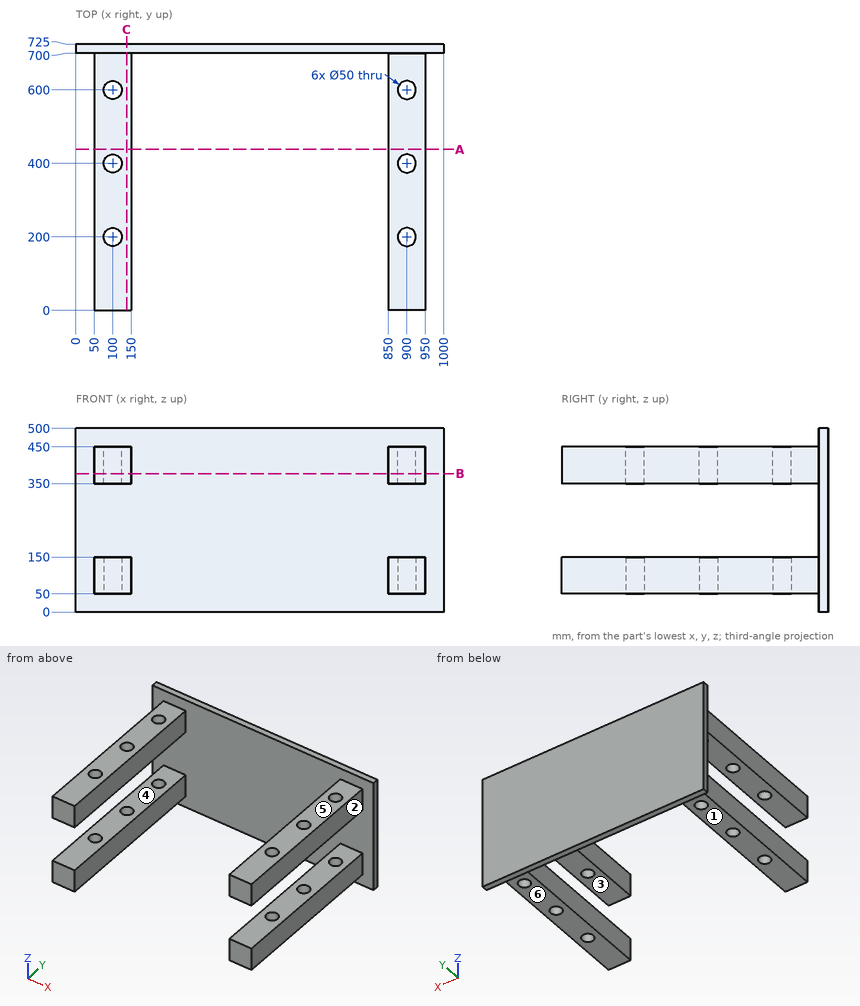
Study the drawing (mm; zero at the part's minimum x, y, z) and answer. A direction names the side the tool comes from. Round coordinates to 2 decimals unless told otherwise and drop trailing zeros. Loops run counter-clockwise (first coordinate to the right, second up) from the corner with the lowest first, then second, coordinate; pieces in that order, holes last.
Q1. Which of the six approach directions +Z, -Z, +X, -X, +Y, -Y give full straight-line access (tool end or side, diameter ignored) to the marked faces 4, 5 and 6?
Q2. Section A-A, the plane y = 438.5 is taken. Determine the outline of the cut face in (x, z).
Q3. Section C-C, the plane x = 137.5 is taken. Determine the outline of the cut face in (y, z), then the cut area to 4 significant figures.
Q4. Find the intervals of material crossed by line 1 (Y direction, x = 100, z = 107); line 2 (Z direction, x = 56.5, y = 387); line 3 (X direction, y = 355.5, z = 414), in increasing order.
Q5. Given pin 1 Ø1 at (x, y) = (109, 493.5) entering from -Z; pin 2 Ø10 at (x, y) = (881, 151) entering from +Z; pin 3 Ø3 at (x, z) = (765.5, 105) entering from -Y, each flat-ended and moving along its own axis, determine where each tip first touches the part or whether it passes through.
Q6. Section B-B, the plane z = 377 is taken. Determine the outline of the cut face in (x, y), then the cut area to 3 significant figures.
Q7. For a pull along Z with two mould halves and no side action, classify the marked faces 1, 2 and 3 as released by +Z, released by -Z, zero draft, split by the parting line, or undercut.
Completed:
1. face 4: +X, -X, -Y
1. face 5: +Z, +X, -X, -Y
1. face 6: -Z, +X, -X, -Y
2. outline: (50, 50) - (150, 50) - (150, 150) - (50, 150) - close; (50, 350) - (150, 350) - (150, 450) - (50, 450) - close; (850, 50) - (950, 50) - (950, 150) - (850, 150) - close; (850, 350) - (950, 350) - (950, 450) - (850, 450) - close
3. outline: (0, 50) - (700, 50) - (700, 0) - (725, 0) - (725, 500) - (700, 500) - (700, 450) - (0, 450) - (0, 350) - (700, 350) - (700, 150) - (0, 150) - close
3. area: 152,500 mm2
4. line 1: y = 0 to 175, 225 to 375, 425 to 575, 625 to 725
4. line 2: z = 50 to 150, 350 to 450
4. line 3: x = 50 to 150, 850 to 950
5. pin 1: stops at z = 50
5. pin 2: stops at z = 450
5. pin 3: stops at y = 700
6. outline: (0, 700) - (50, 700) - (50, 0) - (150, 0) - (150, 700) - (850, 700) - (850, 0) - (950, 0) - (950, 700) - (1000, 700) - (1000, 725) - (0, 725) - close; hole circle Ø50 at (100, 200); hole circle Ø50 at (100, 400); hole circle Ø50 at (100, 600); hole circle Ø50 at (900, 200); hole circle Ø50 at (900, 400); hole circle Ø50 at (900, 600)
6. area: 153,000 mm2
7. face 1: released by -Z
7. face 2: zero draft
7. face 3: undercut
